```python
from build123d import *

# Parameters (mm, degrees)
F0_W     = 53.34
F0_H     = 5.588
F0_H_2   = 27.432
F0_R     = 1.778
F1_DEPTH = 5.08
F2_DEPTH = 42.164
F3_R     = 1.524
F3_R_2   = 11.43
F4_DEPTH = 25.4


with BuildPart() as f1:
    # F0 (on Top) → F1 (new body)
    with BuildSketch(Plane.XY):
        with Locations((26.67, 2.794)):
            Rectangle(F0_W, F0_H)
        with Locations((26.67, 19.304)):
            Rectangle(F0_W, F0_H_2)
        with Locations((2.54, 10.668)):
            Circle(F0_R, mode=Mode.SUBTRACT)
        with Locations((50.8, 10.668)):
            Circle(F0_R, mode=Mode.SUBTRACT)
        with Locations((2.54, 27.94)):
            Circle(F0_R, mode=Mode.SUBTRACT)
        with Locations((50.8, 27.94)):
            Circle(F0_R, mode=Mode.SUBTRACT)
    extrude(amount=-F1_DEPTH)

    # F0 (on Top) → F2 (join)
    with BuildSketch(Plane.XY):
        with Locations((26.67, 2.794)):
            Rectangle(F0_W, F0_H)
    extrude(amount=F2_DEPTH)

    # F3 (on face) → F4 (cut)
    with BuildSketch(Plane.XZ):
        with Locations((11.43, 33.128857)):
            Circle(F3_R)
        with Locations((41.91, 33.128857)):
            Circle(F3_R)
        with Locations((11.43, 9.035143)):
            Circle(F3_R)
        with Locations((41.91, 9.035143)):
            Circle(F3_R)
        with Locations((26.67, 21.082)):
            Circle(F3_R_2)
    extrude(amount=-F4_DEPTH, mode=Mode.SUBTRACT)


solid = f1.part
```
Build history of the part. All positions in model axes, mm. A direction names the side the tool comes from. Coordinates: 2 decimals unless noted, no trailing zeros. Write each loop counter-clockwise with the first axis right and the second up, starting at its lowest first coordinate (ties: lowest second). Pieces come first, ordered by that corner, then holes.
1. 3-axis set-ups, long thin cutter, end or side, ignore diameter. For faces 1 (the flat face through (20, 5.588, 11)), 2 (the cylindrical face through (43.364, 2.755, 9.493)): which of +Z, -Z, +X, -X, +Y, -Y reach the whole face in a straight line?
Answer block:
face 1: +Z, +X, -X, +Y
face 2: +Y, -Y
2. Drill centre lines: probe 1 along Y at (x, z) = (2.54, -1.2); probe 2 along Z at (x, y) = (6, 10); probe 3 along X at (y, z) = (2, 18). Where is each one in solid material? Low to high.
Answer block:
probe 1: y = 0 to 8.89, 12.45 to 26.16, 29.72 to 33.02
probe 2: z = -5.08 to 0
probe 3: x = 0 to 15.66, 37.68 to 53.34
3. Pull direction Z, two halves, no side cores. Call faces 3 (the flat face through (53.34, 5, 11)), 4 (the flat face through (26, 19, 0)), 5 (the cylindrical face through (11.1, 2.75, 31.64)): released by +Z, released by -Z, zero draft, split by the parting line, or undercut.
Answer block:
face 3: zero draft
face 4: released by +Z
face 5: undercut
4. Band-saw the part on B-B, the plane x = 26.67. Give the cut face in (y, z).
Answer block:
outline: (0, -5.08) - (33.02, -5.08) - (33.02, 0) - (5.59, 0) - (5.59, 9.65) - (0, 9.65) - close; (0, 32.51) - (5.59, 32.51) - (5.59, 42.16) - (0, 42.16) - close
5. Band-saw the part on A-A, the plane x = 50.8. Give the cut face in (y, z), and give its area (3 significant figures).
Answer block:
outline: (0, -5.08) - (8.89, -5.08) - (8.89, 0) - (5.59, 0) - (5.59, 42.16) - (0, 42.16) - close; (12.45, -5.08) - (26.16, -5.08) - (26.16, 0) - (12.45, 0) - close; (29.72, -5.08) - (33.02, -5.08) - (33.02, 0) - (29.72, 0) - close
area: 367 mm2
6. Drop flat-ended pins along their axis: pin 1 (2.5 mm diameter, centred on x = 11.43, z = 33.13, fed in from -Y); pin 2 (4 mm diameter, centred on x = 50.8, y = 10.668, fed in from +Z). Give the stop position or say it passes through.
Answer block:
pin 1: passes through
pin 2: stops at z = 0
7. Band-saw the part on D-D, the plane y = 27.94. Give the cut face in (x, z).
Answer block:
outline: (0, -5.08) - (0.76, -5.08) - (0.76, 0) - (0, 0) - close; (4.32, -5.08) - (49.02, -5.08) - (49.02, 0) - (4.32, 0) - close; (52.58, -5.08) - (53.34, -5.08) - (53.34, 0) - (52.58, 0) - close
8. Band-saw the part on C-C, the plane z = 19. Give the cut face in (x, y).
Answer block:
outline: (0, 0) - (15.43, 0) - (15.43, 5.59) - (0, 5.59) - close; (37.91, 0) - (53.34, 0) - (53.34, 5.59) - (37.91, 5.59) - close
